```python
from build123d import *

# Parameters (mm, degrees)
F0_R           = 19.8
F0_R_2         = 16.8
F1_DEPTH       = 25
F2_R           = 19.8
F2_R_2         = 16.8
F3_DEPTH       = 4
F5_DEPTH       = 29
F6_SIZE2       = 55
F6_SIZE        = 15
F6_2_SIZE2     = 55
F6_2_SIZE      = 15
F7_R           = 5
F9_DEPTH       = 25
F10_DEPTH      = 13.8
F10_DEPTH_BACK = 25.8
F11_T4_ANGLE   = 359.64
F11_T10_ANGLE  = 359.64
F11_T16_ANGLE  = 359.64
F11_T22_ANGLE  = 359.64
F12_W          = 8
F12_H          = 8
F13_DEPTH      = 3


# Not quite as in the source:
# - a fillet or chamfer that OpenCascade refuses, or shapes differently, is made with other operations: its cross-section is extruded or revolved along the edge and cut away or added


with BuildPart() as f1:
    # F0 (on Top) → F1 (new body)
    with BuildSketch(Plane.XY):
        Circle(F0_R)
        Circle(F0_R_2, mode=Mode.SUBTRACT)
    extrude(amount=F1_DEPTH)

    # F2 (on face) → F3 (join)
    with BuildSketch(Plane.XY.offset(25)):
        Circle(F2_R)
        Circle(F2_R_2, mode=Mode.SUBTRACT)
        Circle(F2_R_2)
    extrude(amount=F3_DEPTH)

    # F4 (on face) → F5 (join)
    with BuildSketch(Plane.XY.offset(29)):
        with BuildLine():
            Line((-77, -6), (-18.8690222322, -6))
            ThreePointArc((-18.8690222322, -6), (-19.8, 0), (-18.8690222322, 6))
            Line((-18.8690222322, 6), (-77, 6))
            Line((-77, 6), (-77, -6))
        make_face()
        with BuildLine():
            Line((18.8690222322, -6), (77, -6))
            Line((77, -6), (77, 6))
            Line((77, 6), (18.8690222322, 6))
            ThreePointArc((18.8690222322, 6), (19.5658713095, 3.0358985327), (19.8, 0))
            ThreePointArc((19.8, 0), (19.5658713095, -3.0358985327), (18.8690222322, -6))
        make_face()
    extrude(amount=-F5_DEPTH)

    # F6
    f6_edges = [f1.edges().sort_by_distance(p)[0] for p in [
        (77, 0, 0),
    ]]
    f6_side = f1.faces().sort_by_distance((77, 0, 14.5))[0]
    chamfer(f6_edges, length=F6_SIZE, length2=F6_SIZE2, reference=f6_side)

    # F6#2
    f6_2_edges = [f1.edges().sort_by_distance(p)[0] for p in [
        (-77, 0, 0),
    ]]
    f6_2_side = f1.faces().sort_by_distance((-77, 0, 14.5))[0]
    chamfer(f6_2_edges, length=F6_2_SIZE, length2=F6_2_SIZE2, reference=f6_2_side)

    # F7 (call 1 of 4: OpenCascade refuses the feature's edges together)
    f7_edges = [f1.edges().sort_by_distance(p)[0] for p in [
        (-18.869022, 6, 14.5),
    ]]
    fillet(f7_edges, radius=F7_R)

    # F7#2 (call 2 of 4)
    f7_2_edges = [f1.edges().sort_by_distance(p)[0] for p in [
        (18.869022, 6, 14.5),
    ]]
    fillet(f7_2_edges, radius=F7_R)

    # F7#3 (call 3 of 4)
    f7_3_edges = [f1.edges().sort_by_distance(p)[0] for p in [
        (-18.869022, -6, 14.5),
    ]]
    fillet(f7_3_edges, radius=F7_R)

    # F7#4 (call 4 of 4)
    f7_4_edges = [f1.edges().sort_by_distance(p)[0] for p in [
        (18.869022, -6, 14.5),
    ]]
    fillet(f7_4_edges, radius=F7_R)

    # F8 (on face) → F9 (cut)
    with BuildSketch(Plane.XZ.offset(6)):
        with BuildLine():
            ThreePointArc((68, 29), (70.8284271247, 27.8284271247), (72, 25))
            Line((72, 25), (72, 29))
            Line((72, 29), (68, 29))
        make_face()
        with BuildLine():
            Line((64, 29), (64, 25))
            ThreePointArc((64, 25), (65.1715728753, 27.8284271247), (68, 29))
            Line((68, 29), (64, 29))
        make_face()
        with BuildLine():
            ThreePointArc((68, 29), (65.1715728753, 27.8284271247), (64, 25))
            ThreePointArc((64, 25), (68, 21), (72, 25))
            ThreePointArc((72, 25), (70.8284271247, 27.8284271247), (68, 29))
        make_face()
        with BuildLine():
            Line((-72, 29), (-72, 25))
            ThreePointArc((-72, 25), (-70.8284271247, 27.8284271247), (-68, 29))
            Line((-68, 29), (-72, 29))
        make_face()
        with BuildLine():
            ThreePointArc((-68, 29), (-65.1715728753, 27.8284271247), (-64, 25))
            Line((-64, 25), (-64, 29))
            Line((-64, 29), (-68, 29))
        make_face()
        with BuildLine():
            ThreePointArc((-68, 29), (-70.8284271247, 27.8284271247), (-72, 25))
            ThreePointArc((-72, 25), (-68, 21), (-64, 25))
            ThreePointArc((-64, 25), (-65.1715728753, 27.8284271247), (-68, 29))
        make_face()
    extrude(amount=-F9_DEPTH, mode=Mode.SUBTRACT)

    # F8 (on face) → F10 (join, two sides)
    with BuildSketch(Plane.XZ.offset(6)) as f10_sk:
        with BuildLine():
            ThreePointArc((-64, 25), (-68, 21), (-72, 25))
            Line((-72, 25), (-72, 29))
            Line((-72, 29), (-73.7445626465, 29))
            ThreePointArc((-73.7445626465, 29), (-70.0961943462, 18.3212299588), (-61, 25))
            ThreePointArc((-61, 25), (-61.3212299588, 27.0961943462), (-62.2554373535, 29))
            Line((-62.2554373535, 29), (-64, 29))
            Line((-64, 29), (-64, 25))
        make_face()
        with BuildLine():
            ThreePointArc((72, 25), (68, 21), (64, 25))
            Line((64, 25), (64, 29))
            Line((64, 29), (62.2554373535, 29))
            ThreePointArc((62.2554373535, 29), (65.9038056538, 18.3212299588), (75, 25))
            ThreePointArc((75, 25), (74.6787700412, 27.0961943462), (73.7445626465, 29))
            Line((73.7445626465, 29), (72, 29))
            Line((72, 29), (72, 25))
        make_face()
    extrude(amount=F10_DEPTH)
    extrude(f10_sk.sketch, amount=-F10_DEPTH_BACK)

    # F11: fillet of radius 5 on 4 edges, made by hand


with BuildPart() as f11_tool2:
    # F11_s3 → F11_t4 (revolve)
    with BuildSketch(Plane(origin=(67.9207895695, 0, -0.2133801555), x_dir=(0, 1, 0), z_dir=(-0.9999950652, 0, 0.0031415875))):
        with BuildLine():
            ThreePointArc((6, -37.2135045791), (7.4644660941, -33.6779706732), (11, -32.2135045791))
            Line((11, -32.2135045791), (6, -32.2135045791))
            Line((6, -32.2135045791), (6, -37.2135045791))
        make_face()
    revolve(axis=Axis((68, 6, 25), (0, 1, 0)), revolution_arc=F11_T4_ANGLE)

    split(bisect_by=Plane.XY.offset(29), keep=Keep.BOTTOM)

    split(bisect_by=Plane.YZ.offset(77), keep=Keep.BOTTOM)


with BuildPart() as f1_1:
    add(f1.part)

    # F11_t1: union F11_tool2
    add(f11_tool2.part)


with BuildPart() as f11_tool8:
    # F11_s9 → F11_t10 (revolve)
    with BuildSketch(Plane(origin=(67.9207895695, 0, -0.2133801555), x_dir=(0, 1, 0), z_dir=(-0.9999950652, 0, 0.0031415875))):
        with BuildLine():
            ThreePointArc((-11, -32.2135045791), (-7.4644660941, -33.6779706732), (-6, -37.2135045791))
            Line((-6, -37.2135045791), (-6, -32.2135045791))
            Line((-6, -32.2135045791), (-11, -32.2135045791))
        make_face()
    revolve(axis=Axis((68, -6, 25), (0, 1, 0)), revolution_arc=F11_T10_ANGLE)

    split(bisect_by=Plane.XY.offset(29), keep=Keep.BOTTOM)

    split(bisect_by=Plane.YZ.offset(77), keep=Keep.BOTTOM)


with BuildPart() as f1_2:
    add(f1_1.part)

    # F11_t7: union F11_tool8
    add(f11_tool8.part)


with BuildPart() as f11_tool14:
    # F11_s15 → F11_t16 (revolve)
    with BuildSketch(Plane(origin=(-68.0778681687, 0, 0.2138736341), x_dir=(0, 1, 0), z_dir=(-0.9999950652, 0, 0.0031415875))):
        with BuildLine():
            ThreePointArc((11, -31.786248681), (7.4644660941, -33.2507147751), (6, -36.786248681))
            Line((6, -36.786248681), (6, -31.786248681))
            Line((6, -31.786248681), (11, -31.786248681))
        make_face()
    revolve(axis=Axis((-68, 6, 25), (0, 1, 0)), revolution_arc=F11_T16_ANGLE)

    split(bisect_by=Plane.XY.offset(29), keep=Keep.BOTTOM)

    split(bisect_by=Plane.YZ.offset(-77), keep=Keep.TOP)


with BuildPart() as f1_3:
    add(f1_2.part)

    # F11_t13: union F11_tool14
    add(f11_tool14.part)


with BuildPart() as f11_tool20:
    # F11_s21 → F11_t22 (revolve)
    with BuildSketch(Plane(origin=(-68.0778681687, 0, 0.2138736341), x_dir=(0, 1, 0), z_dir=(-0.9999950652, 0, 0.0031415875))):
        with BuildLine():
            ThreePointArc((-6, -36.786248681), (-7.4644660941, -33.2507147751), (-11, -31.786248681))
            Line((-11, -31.786248681), (-6, -31.786248681))
            Line((-6, -31.786248681), (-6, -36.786248681))
        make_face()
    revolve(axis=Axis((-68, -6, 25), (0, 1, 0)), revolution_arc=F11_T22_ANGLE)

    split(bisect_by=Plane.XY.offset(29), keep=Keep.BOTTOM)

    split(bisect_by=Plane.YZ.offset(-77), keep=Keep.TOP)


with BuildPart() as f1_4:
    add(f1_3.part)

    # F11_t19: union F11_tool20
    add(f11_tool20.part)

    # F12 (on face) → F13 (join)
    with BuildSketch(Plane.XZ.offset(19.8)):
        with Locations((68, 25)):
            Rectangle(F12_W, F12_H)
        with BuildLine():
            Line((-64, 29), (-72, 29))
            Line((-72, 29), (-72, 25))
            ThreePointArc((-72, 25), (-70.8284271247, 22.1715728753), (-68, 21))
            ThreePointArc((-68, 21), (-65.1715728753, 22.1715728753), (-64, 25))
            Line((-64, 25), (-64, 29))
        make_face()
        with BuildLine():
            Line((-64, 21), (-64, 25))
            ThreePointArc((-64, 25), (-65.1715728753, 22.1715728753), (-68, 21))
            Line((-68, 21), (-64, 21))
        make_face()
        with BuildLine():
            ThreePointArc((-68, 21), (-70.8284271247, 22.1715728753), (-72, 25))
            Line((-72, 25), (-72, 21))
            Line((-72, 21), (-68, 21))
        make_face()
    extrude(amount=-F13_DEPTH)


solid = f1_4.part
```
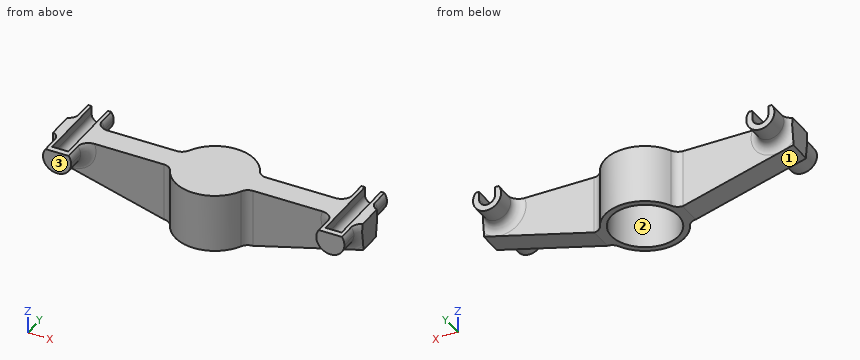
For this review, take the finished solid that the model builds, in its own axes (mm). Face numbers are marked on the shaded views. Give positions to 0.01 mm unless a question says otherwise; leave off trailing zeros. Write each loop counter-clockwise with the first axis right and the second up, starting at its lowest first coordinate (ties: lowest second). Pieces come first, ordered by that corner, then holes. Notation, with made-up numbers: M -21,46.5 L 37,46.5 A25 cw 37,74.5 Z; hole C -16,-37 d10. An arc over 180 degrees is marked long. Answer as CSV lines item,"result".
1. Wall thickness on line 1 (Y direction, x = 0, z = 19.5); line 2 (X direction, y = 4.5, z = 27.25); line 3 (X direction, y = -9.5, z = 24): over which ranges is each line inside the solid? List them lowest first.
Findings:
line 1,"y = -19.8 to -16.8, 16.8 to 19.8"
line 2,"x = -77 to -72, -64 to 64, 72 to 77"
line 3,"x = -75.16 to -71.87, -64.13 to -60.84, -17.37 to -13.86, 13.86 to 17.37, 60.84 to 64.13, 71.87 to 75.16"
2. Consider section A-A, the plane x = 0. Write out the cut boundary in (y, z), then the cut area to 3 significant figures.
Findings:
outline,"M -19.8,0 L -16.8,0 L -16.8,25 L 16.8,25 L 16.8,0 L 19.8,0 L 19.8,29 L -19.8,29 Z"
area,"308 mm2"
3. Consider section D-D, the plane x = -51. Write out the cut boundary in (y, z), then the cut area to 3 significant figures.
Findings:
outline,"M -6,7.91 L 6,7.91 L 6,29 L -6,29 Z"
area,"253 mm2"
4. Consider section B-B, the plane y = 0. Write out the cut boundary in (x, z), then the cut area to 3 significant figures.
Findings:
outline,"M -77,15 L -22,0 L -16.8,0 L -16.8,25 L 16.8,25 L 16.8,0 L 22,0 L 77,15 L 77,29 L 72,29 L 72,25 A4 cw 64,25 L 64,29 L -64,29 L -64,25 A4 cw -72,25 L -72,29 L -77,29 Z"
area,"2,690 mm2"
5. For pin 1 (10 mm diameter, centred on y = -14.5, z = 14.5, fed in from -X); pin 2 (2 mm diameter, centred on y = 10, z = 26.5, fed in from -X); pin 3 (2.5 mm diameter, centred on x = -67.5, z = 26.5, fed in from +Y), all flat-tipped, find the tip position at first contact; note any pin that passes through.
Findings:
pin 1,"stops at x = -72.33"
pin 2,"stops at x = -75.3"
pin 3,"stops at y = -16.8"
6. Draft analysis for pull direction X (two halves, no side actions). For the marked faces 1, 2 and 3, state which applies: +X half, -X half, draft (parallel to the pull), parting line (faces both ways), or undercut.
Findings:
face 1,"-X half"
face 2,"undercut"
face 3,"draft"
7. Consider section C-C, the plane x = -68. Write out the cut boundary in (y, z), then the cut area to 3 significant figures.
Findings:
outline,"M -19.8,18 L -11,18 A5 cw -6,13 L -6,12.55 L 6,12.55 L 6,13 A5 cw 11,18 L 19.8,18 L 19.8,21 L -16.8,21 L -16.8,29 L -19.8,29 Z"
area,"219 mm2"
